Here's how the part is built. I have some questions about the finished solid (model axes, mm). A direction names the side the tool comes from. Coordinates: 2 decimals unless noted, no trailing zeros. Order: outer loops, then holes, each group sorted by start corner. A loop starts at its lowest first (then second) coordinate and runs counter-clockwise, first axis right, second up. Notation, with made-up numbers: (41, 53.25) - (80, 53.25) arc R19 ccw to (80, 90.25) - close; hole circle Ø2 at (49, -36.75). An arc over 180 degrees is marked (long way). Answer as CSV lines item,"result". Start each with the question number.
Item 1: I need wall thicknesses on line 1 (Y direction, x = 14.92, z = 0.7); line 2 (X direction, y = 21.11, z = 0.4); line 3 (Z direction, x = 16, y = 19). Which ranges of each line are inside material? Lowest first, please.
Item 2: Imagine slicing it at B-B on y = 21.11. List the corners of the cut face in (x, z) for me.
Item 3: I'm going to push flat-ended pins straight in: pin 1 (1.5 mm diameter, centred on x = 1.5, z = 3, fed in from -Y); pin 2 (10 mm diameter, centred on x = 12.5, y = 13, fed in from +Z); pin 3 (0.9 mm diameter, centred on y = 7.5, z = 2, fed in from +X). Where does each tip first touch, or does it pass through?
Item 4: Imagine slicing it at D-D on x = 4.25. List the corners of the cut face in (y, z) for me, and give its area (3 significant figures).
Item 5: On a 3-axis mill with a long thin cutter (end or side, diameter ignored), from which of +Z, -Z, +X, -X, +Y, -Y can I reach the whole of each face in a straight line? I mean faces 4 (the face through (3, 2.476, 2)), 5 (the face through (3, 12.283, 2)), 6 (the face through (8.7, 0, 0.5)). Say none if no direction works.
Item 6: We'd pull the mould along X, two halves only. Please class faces 1 (the face through (9, 12, 0)), 2 (the face through (13.52, 21.17, 0.49)), 3 (the face through (5.073, 7, 2)): pulls with the +X half, pulls with the -X half, needs draft (parallel to the pull), parting line crosses it, or undercut.
Item 7: Imagine slicing it at C-C on z = 0.7. List the corners of the cut face in (x, y) for me, and give its area (3 significant figures).
Item 8: Imagine slicing it at A-A on x = 14.92. List the corners of the cut face in (y, z) for me, and give its area (3 significant figures).
from build123d import *

# Parameters (mm, degrees)
F0_W     = 17.62
F0_H     = 24
F2_DEPTH = 1
F1_R     = 1.4
F3_DEPTH = 3
F4_W     = 5.072871
F4_H     = 9.807147
F5_DEPTH = 3


with BuildPart() as f2:
    # F0 (on Top) → F2 (new body)
    with BuildSketch(Plane.XY):
        with Locations((8.81, 12)):
            Rectangle(F0_W, F0_H)
    extrude(amount=F2_DEPTH)

    # F1 (on face) → F3 (cut)
    with BuildSketch(Plane.XY):
        with Locations((14.92, 2.7)):
            Circle(F1_R)
        with Locations((14.92, 21.11)):
            Circle(F1_R)
    extrude(amount=F3_DEPTH, mode=Mode.SUBTRACT)

    # F4 (on face) → F5 (join)
    with BuildSketch(Plane.XY.offset(1)):
        with Locations((2.536436, 7.37925)):
            Rectangle(F4_W, F4_H)
    extrude(amount=F5_DEPTH)


solid = f2.part
Responses:
1,line 1,"y = 0 to 1.3, 4.1 to 19.71, 22.51 to 24"
1,line 2,"x = 0 to 13.52, 16.32 to 17.62"
1,line 3,"z = 0 to 1"
2,outline,"(0, 0) - (13.52, 0) - (13.52, 1) - (0, 1) - close; (16.32, 0) - (17.62, 0) - (17.62, 1) - (16.32, 1) - close"
3,pin 1,"stops at y = 2.48"
3,pin 2,"stops at z = 1"
3,pin 3,"stops at x = 5.07"
4,outline,"(0, 0) - (24, 0) - (24, 1) - (12.28, 1) - (12.28, 4) - (2.48, 4) - (2.48, 1) - (0, 1) - close"
4,area,"53.4 mm^2"
5,face 4,"+Z, +X, -X, -Y"
5,face 5,"+Z, +X, -X, +Y"
5,face 6,"+Z, -Z, +X, -X, -Y"
6,face 1,"needs draft"
6,face 2,"undercut"
6,face 3,"pulls with the +X half"
7,outline,"(0, 0) - (17.62, 0) - (17.62, 24) - (0, 24) - close; hole circle Ø2.8 at (14.92, 2.7); hole circle Ø2.8 at (14.92, 21.11)"
7,area,"411 mm^2"
8,outline,"(0, 0) - (1.3, 0) - (1.3, 1) - (0, 1) - close; (4.1, 0) - (19.71, 0) - (19.71, 1) - (4.1, 1) - close; (22.51, 0) - (24, 0) - (24, 1) - (22.51, 1) - close"
8,area,"18.4 mm^2"
